Input: part model. Units: mm. Frame: model coordinates. A direction names the side the tool comes from. Round coordinates to 2 decimals unless told otherwise and drop trailing zeros. Write each loop counter-clockwise with the first axis right and the second up, starting at its lowest first coordinate (ties: lowest second). Pieces come first, ordered by that corner, then holes. Notation, with made-up numbers: (8.5, 73) -> (60.5, 73) arc R21 cw to (60.5, 92) -> close; hole circle Ø7 at (73.5, 50). An arc over 180 degrees is marked (long way). Use CSV: the item, a comma, the result in double quotes.
Autodesk Inventor part; units mm, degrees
ref_plane "YZ Plane" through (0, 0, 0) normal (1, 0, 0) x (0, 1, 0)
ref_plane "XZ Plane" through (0, 0, 0) normal (0, 1, 0) x (-1, 0, 0)
ref_plane "XY Plane" through (0, 0, 0) normal (0, 0, 1) x (1, 0, 0)
sketch "Sketch1" plane through (0, 0, 0) normal (0, 0, 1) x (1, 0, 0)
  line L0 (-2.8575, 0) -> (-2.8575, -25.4)
  line L1 (-2.8575, -25.4) -> (-6.0325, -25.4)
  line L2 (-6.0325, -25.4) -> (-6.0325, 6.35)
  line L3 (2.8575, 0) -> (2.8575, -25.4)
  line L4 (2.8575, -25.4) -> (6.0325, -25.4)
  line L5 (6.0325, -25.4) -> (6.0325, 6.35)
  line L6 (-6.0325, 6.35) -> (6.0325, 6.35)
  line L7 (2.8575, 0) -> (-2.8575, 0)
  point P0 (0, 0)
  point P1 (0, 0)
  dimension "d0" = 5.715
  dimension "d1" = 3.175
  dimension "d2" = 25.4
  dimension "d3" = 31.75
extrude "Extrusion1" add sketch "Sketch1" along normal blind 88.9
sketch "Sketch2" plane through (-6.0325, -25.4, 0) normal (-1, 0, 0) x (0, 0, 1)
  line L0 (22.225, 31.75) -> (66.675, 31.75)
  line L1 (66.675, 31.75) -> (66.675, 25.4)
  line L2 (66.675, 25.4) -> (22.225, 25.4)
  line L3 (22.225, 25.4) -> (22.225, 31.75)
  line L4 (0, 31.75) -> (88.9, 31.75)
  point P0 (0, 25.4)
  point P1 (44.45, 31.75)
  dimension "d9" = 6.35
  dimension "d10" = 44.45
extrude "Extrusion2" add sketch "Sketch2" along normal blind 31.115
sketch "Sketch3" plane through (-6.0325, 6.35, 0) normal (0, 1, 0) x (1, 0, 0)
  line L0 (12.065, 0) -> (12.065, -88.9)
  line L1 (12.065, -22.225) -> (5.715, -22.225)
  line L2 (5.715, -22.225) -> (5.715, -66.675)
  line L3 (5.715, -66.675) -> (12.065, -66.675)
  line L4 (12.065, -66.675) -> (12.065, -22.225)
  line L5 (0, -22.225) -> (-31.115, -22.225)
  line L6 (0, -66.675) -> (-31.115, -66.675)
  point P0 (6.0325, 0)
  dimension "d13" = 6.35
extrude "Extrusion3" add sketch "Sketch3" along normal blind 50.8
sketch "Sketch4" plane through (-0.3175, 57.15, 22.225) normal (-1, 0, 0) x (0, 0, 1)
  line L0 (0, -50.8) -> (0, 0)
  line L1 (44.45, 0) -> (0, 0)
  line L2 (0, 0) -> (0, -6.35)
  line L3 (0, -6.35) -> (44.45, -6.35)
  line L4 (44.45, -6.35) -> (44.45, 0)
  line L5 (0, 0) -> (44.45, 0)
  line L6 (44.45, -50.8) -> (44.45, 0)
  point P0 (-22.225, -57.15)
  point P1 (44.45, -45.72)
  dimension "d17" = 6.35
extrude "Extrusion4" add sketch "Sketch4" along normal up to surface (36.83 mm away)
chamfer "Chamfer1" distance 5.08 angle 45 1 edges at (-0.3175, 50.8, 44.45)
chamfer "Chamfer2" distance 5.08 angle 45 1 edges at (-0.3175, 6.35, 44.45)
chamfer "Chamfer3" distance 5.08 angle 45 1 edges at (-6.0325, 0, 44.45)
sketch "Sketch5" plane through (6.0325, -25.4, 0) normal (1, 0, 0) x (0, 0, -1)
  line L0 (-88.9, 0) -> (-88.9, 31.75)
  line L1 (0, 31.75) -> (0, 0)
  line L2 (0, 0) -> (-88.9, 0)
  point P0 (0, 25.4)
  point P1 (-69.85, 12.7)
  point P2 (-19.05, 12.7)
  dimension "d29" = 19.05
  dimension "d30" = 19.05
  dimension "d31" = 12.7
  dimension "d32" = 12.7
hole "Hole1" at (6.0325, -12.7, 69.85) at (6.0325, -12.7, 19.05) direction (-1, 0, 0) diameter 6.35 end through all
sketch "Sketch6" plane through (6.0325, -25.4, 0) normal (1, 0, 0) x (0, 0, -1)
  line L0 (-28.575, 6.35) -> (-60.325, 6.35)
  line L1 (-60.325, 6.35) -> (-60.325, 19.05)
  line L2 (-60.325, 19.05) -> (-28.575, 19.05)
  line L3 (-28.575, 19.05) -> (-28.575, 6.35)
  circle A0 centre (-69.85, 12.7) radius 3.175
  circle A1 centre (-19.05, 12.7) radius 3.175
  line L4 (0, 0) -> (-88.9, 0)
  point P0 (0, 25.4)
  dimension "d40" = 31.75
  dimension "d41" = 50.8
  dimension "d42" = 9.525
  dimension "d43" = 12.7
  dimension "d44" = 6.35
extrude "Extrusion5" cut sketch "Sketch6" against normal blind 50.8 contours L0 L1 L2 L3
sketch "Sketch7" plane through (-6.0325, 57.15, 0) normal (0, 1, 0) x (1, 0, 0)
  circle A0 centre (-15.5575, -44.45) radius 6.35
  line L0 (-31.115, -22.225) -> (-31.115, -66.675)
  line L1 (0, -22.225) -> (0, -66.675)
  line L2 (12.065, -66.675) -> (-31.115, -66.675)
  line L3 (12.065, -22.225) -> (-31.115, -22.225)
  point P0 (6.0325, 0)
  dimension "d47" = 15.5575
  dimension "d48" = 31.115
  dimension "d49" = 44.45
  dimension "d50" = 22.225
  dimension "d51" = 12.7
extrude "Extrusion6" cut sketch "Sketch7" against normal blind 101.6 contours A0
sketch "Sketch8" plane through (6.0325, -25.4, 0) normal (1, 0, 0) x (0, 0, -1)
  line L0 (-66.675, 31.75) -> (-66.675, 82.55)
  line L1 (-66.675, 82.55) -> (-22.225, 82.55)
  point P0 (0, 25.4)
  point P1 (-53.975, 57.15)
  point P2 (-34.925, 57.15)
  dimension "d54" = 19.05
  dimension "d55" = 12.7
  dimension "d56" = 25.4
  dimension "d57" = 50.8
  dimension "d58" = 25.4
hole "Hole2" at (6.0325, 31.75, 53.975) at (6.0325, 31.75, 34.925) direction (-1, 0, 0) diameter 6.35 end through all
equation "\"d47\" = 0.5 * d48"
equation "\"d50\" = 0.5 * d49"
properties part number "Suspension Frame 3.0"
Item 1: Set-up query: faces 5 (the face through (4, -13, 60.325)), 6 (the face through (-30, 0, 45)), 7 (the face through (-18, 50.8, 39)). Return all of +Z, -Z, +X, -X, +Y, -Y with unobstructed straight access to the full face (end or side cutting, diameter ignored); none if empty.
Worked answers:
face 5,"+X, -X"
face 6,"+Z, -Z, -X, -Y"
face 7,"+Z, -Z, -X"
Item 2: Section query D-D on x = -21.59. Return the cut outline in (y, z) (3 decimals), plus the area to 3 significant figures.
Worked answers:
outline,"(0, 22.225) -> (6.35, 22.225) -> (6.35, 38.1) -> (0, 38.1) -> close; (0, 50.8) -> (6.35, 50.8) -> (6.35, 66.675) -> (0, 66.675) -> close; (50.8, 22.225) -> (57.15, 22.225) -> (57.15, 38.1) -> (50.8, 38.1) -> close; (50.8, 50.8) -> (57.15, 50.8) -> (57.15, 66.675) -> (50.8, 66.675) -> close"
area,"403 mm²"
Item 3: First-contact query: pin 1 Ø12.5 at (x, y) = (-14, 1) entering from +Z (3 decimals); pin 2 Ø12 at (x, y) = (-2, 21) entering from -Z (3 decimals); pin 3 Ø20.5 at (y, z) = (-16, 34.5) entering from -X. Flat tips, straight axial feed; report the tip coordinate or a pass-through.
Worked answers:
pin 1,"stops at z = 66.675"
pin 2,"stops at z = 22.225"
pin 3,"stops at x = -6.03"
Item 4: Line query: line 1 (Z direction, x = 4.2, y = -12.7) (3 decimals); line 2 (Z direction, x = 3.5, y = 31.75) (3 decimals); line 3 (X direction, y = -20.5, z = 81). Output: solid intervals per line, ascending.
Worked answers:
line 1,"z = 0 to 15.875, 22.225 to 28.575, 60.325 to 66.675, 73.025 to 88.9"
line 2,"z = 22.225 to 31.75, 38.1 to 50.8, 57.15 to 66.675"
line 3,"x = -6.03 to -2.86, 2.86 to 6.03"
Item 5: Pull-direction query (Z, two-part tool) for faces 1 (the face through (4, -6, 0)), 2 (the face through (2.813, 33.682, 56.495)), 3 (the face through (4, -19.05, 44)), 4 (the face through (-2.8, 48.2, 44.1)); classes: +Z half, -Z half, draft (parallel to the pull), parting line (faces both ways), or undercut.
Worked answers:
face 1,"-Z half"
face 2,"undercut"
face 3,"undercut"
face 4,"draft"
Item 6: Section query A-A on y = -12.7. Give the number of separate pieces and of enclosed holes in the cut face, plus the area to 3 significant figures.
Worked answers:
separate pieces,"8"
enclosed holes,"0"
area,"282 mm²"
